from build123d import *

# Parameters (mm, degrees)
F0_W     = 63.5
F0_H     = 63.5
F0_W_2   = 50.8
F0_H_2   = 50.8
F1_DEPTH = 165.1
F3_R     = 6.477
F4_DEPTH = 25.4
F6_DEPTH = 25.4
F7_R     = 6.35
F8_DEPTH = 63.501


# Not quite as in the source:
# - ends of sketch curves that miss each other by under 0.0002 mm in the source are joined


with BuildPart() as f1:
    # F0 (on Top) → F1 (new body, symmetric)
    with BuildSketch(Plane.XY):
        Rectangle(F0_W, F0_H)
        Rectangle(F0_W_2, F0_H_2, mode=Mode.SUBTRACT)
    extrude(amount=F1_DEPTH, both=True)

    # F3 (on face) → F4 (cut)
    with BuildSketch(Plane.YZ.offset(31.75)):
        with Locations((0, 146.05)):
            Circle(F3_R)
        with BuildLine():
            ThreePointArc((10.1385245046, 129.1766616857), (14.6288058895, 132.8781640138), (17.8406687878, 137.7307595176))
            ThreePointArc((17.8406687878, 137.7307595176), (19.4934269332, 143.3103775076), (19.4426449846, 149.1294124443))
            ThreePointArc((19.4426449846, 149.1294124443), (15.0835370951, 152.2964897102), (11.9164598293, 147.9373818207))
            ThreePointArc((11.9164598293, 147.9373818207), (11.9475842494, 144.3708765369), (10.9346034506, 140.9511106721))
            ThreePointArc((10.9346034506, 140.9511106721), (8.9660423194, 137.9769392343), (6.2139343738, 135.708276517))
            ThreePointArc((6.2139343738, 135.708276517), (4.9104220235, 130.4801740359), (10.1385245046, 129.1766616857))
        make_face()
        with BuildLine():
            ThreePointArc((-10.1385245046, 129.1766616857), (-4.9104220235, 130.4801740359), (-6.2139343738, 135.708276517))
            ThreePointArc((-6.2139343738, 135.708276517), (-8.9660423194, 137.9769392343), (-10.9346034506, 140.9511106721))
            ThreePointArc((-10.9346034506, 140.9511106721), (-11.9475842494, 144.3708765369), (-11.9164598293, 147.9373818207))
            ThreePointArc((-11.9164598293, 147.9373818207), (-15.0835370951, 152.2964897102), (-19.4426449846, 149.1294124443))
            ThreePointArc((-19.4426449846, 149.1294124443), (-19.4934269332, 143.3103775076), (-17.8406687878, 137.7307595176))
            ThreePointArc((-17.8406687878, 137.7307595176), (-14.6288058895, 132.8781640138), (-10.1385245046, 129.1766616857))
        make_face()
    extrude(amount=-F4_DEPTH, mode=Mode.SUBTRACT)

    # F5 (on face) → F6 (cut)
    with BuildSketch(Plane(origin=(-31.75, 0, 0), x_dir=(0, -1, 0), z_dir=(-1, 0, 0))):
        with BuildLine():
            ThreePointArc((-3.1401119103, 140.3850881569), (3.2873259769, 140.4692279278), (6.477, 146.05))
            ThreePointArc((6.477, 146.05), (-3.2873259769, 151.6307720722), (-3.1401119103, 140.3850881569))
        make_face()
        with BuildLine():
            ThreePointArc((-5.7913527214, 132.1654121492), (-6.0549491708, 133.1322727306), (-6.7727903948, 133.8315626913))
            ThreePointArc((-6.7727903948, 133.8315626913), (-9.3377562721, 131.1985515677), (-5.7913527214, 132.1654121492))
        make_face()
        with BuildLine():
            ThreePointArc((3.1226517792, 134.3961049058), (0.4285749428, 129.7298269458), (5.0948529028, 127.0357501095))
            ThreePointArc((5.0948529028, 127.0357501095), (17.8406687878, 137.7307595176), (17.8406687878, 154.3692404824))
            ThreePointArc((17.8406687878, 154.3692404824), (12.777460542, 156.2120975737), (10.9346034506, 151.1488893279))
            ThreePointArc((10.9346034506, 151.1488893279), (10.9346034506, 140.9511106721), (3.1226517792, 134.3961049058))
        make_face()
    extrude(amount=-F6_DEPTH, mode=Mode.SUBTRACT)

    # F7 (on face) → F8 (cut, through all)
    with BuildSketch(Plane.YZ.offset(31.75)):
        with BuildLine():
            ThreePointArc((-8.89, 107.949999693), (-15.239999693, 101.6), (-8.89, 95.250000307))
            ThreePointArc((-8.89, 95.250000307), (3.81, 82.55), (-8.89, 69.85))
            ThreePointArc((-8.89, 69.85), (-15.239999693, 63.5), (-8.89, 57.150000307))
            ThreePointArc((-8.89, 57.150000307), (16.509999693, 82.55), (-8.89, 107.949999693))
        make_face()
        with BuildLine():
            ThreePointArc((8.89, 3.07e-07), (15.239999693, 6.35), (8.89, 12.699999693))
            ThreePointArc((8.89, 12.699999693), (-3.81, 25.4), (8.89, 38.1))
            ThreePointArc((8.89, 38.1), (15.24, 44.45), (8.89, 50.8))
            ThreePointArc((8.89, 50.8), (-16.509999693, 25.4), (8.89, 3.07e-07))
        make_face()
        with BuildLine():
            ThreePointArc((-8.89, -6.350000307), (-15.239999693, -12.7), (-8.89, -19.049999693))
            ThreePointArc((-8.89, -19.049999693), (3.81, -31.75), (-8.89, -44.45))
            ThreePointArc((-8.89, -44.45), (-15.239999693, -50.8), (-8.89, -57.149999693))
            ThreePointArc((-8.89, -57.149999693), (16.509999693, -31.75), (-8.89, -6.350000307))
        make_face()
        with BuildLine():
            ThreePointArc((8.89, -114.299999693), (15.239999693, -107.95), (8.89, -101.600000307))
            ThreePointArc((8.89, -101.600000307), (-3.81, -88.9), (8.89, -76.2))
            ThreePointArc((8.89, -76.2), (15.24, -69.85), (8.89, -63.5))
            ThreePointArc((8.89, -63.5), (-16.509999693, -88.9), (8.89, -114.299999693))
        make_face()
        with Locations((-8.89, 82.55)):
            Circle(F7_R)
        with Locations((8.89, 25.4)):
            Circle(F7_R)
        with Locations((8.89, -88.9)):
            Circle(F7_R)
        with Locations((-8.89, -31.75)):
            Circle(F7_R)
    extrude(amount=-F8_DEPTH, mode=Mode.SUBTRACT)


solid = f1.part
Geometry: final body of the model. Coordinates: model frame, mm. A direction names the side the tool comes from. Coordinates: 2 decimals unless noted, no trailing zeros. Loops run counter-clockwise (first coordinate to the right, second up) from the corner with the lowest first, then second, coordinate; pieces in that order, holes last. Notation, with made-up numbers: (69, -17.75) - (97, -17.75) arc R28 cw to (97, 19.25) - close; hole circle Ø5 at (59.25, -18). An arc over 180 degrees is marked (long way). One line per question, with ' | ' between items. Start each with the question number.
(1) Draft query along Z for faces 1 (the flat face through (25.4, -6, 2)), 2 (the flat face through (-29, 0, -165.1)), 3 (the cylindrical face through (-28.53, -15.24, -12.56)). Return one class per face: +Z half, -Z half, draft (parallel to the pull), parting line (faces both ways), or undercut.
(2) Cut plane B-B on x = 22. Output: boundary loops of the cut face in (y, z).
(3) Cut plane D-D on z = -106.5. Output: boundary loops of the cut face in (x, y), and give its area (3 significant figures).
(4) Reachability of faces 4 (the cylindrical face through (-28.619, -12.854, 156.247)), 5 (the flat face through (0, -31.75, 2)), 6 (the cylindrical face through (28.619, -3.807, -89.179)) from +Z, -Z, +X, -X, +Y, -Y: full face, straight path, thin tool, end or side. Return the list, or none.
(5) Cut plane A-A on z = 82.55. Output: boundary loops of the cut face in (x, y).
(6) Ray query, L1, parallel to Y at x = -29, z = 146; L2, parallel to X at y = 2, z = -83.5. Return the intervals inside material, ascending. Write a range as from..to.
Here are the results:
1) face 1: draft | face 2: -Z half | face 3: undercut
2) outline: (-31.75, -165.1) - (-25.4, -165.1) - (-25.4, 165.1) - (-31.75, 165.1) - close; (25.4, -165.1) - (31.75, -165.1) - (31.75, 165.1) - (25.4, 165.1) - close
3) outline: (-31.75, -31.75) - (31.75, -31.75) - (31.75, -9.42) - (25.4, -9.42) - (25.4, -25.4) - (-25.4, -25.4) - (-25.4, -9.42) - (-31.75, -9.42) - close; (-31.75, 15.07) - (-25.4, 15.07) - (-25.4, 25.4) - (25.4, 25.4) - (25.4, 15.07) - (31.75, 15.07) - (31.75, 31.75) - (-31.75, 31.75) - close | area: 1,140 mm²
4) face 4: -X | face 5: +Z, -Z, +X, -X, -Y | face 6: +X, -X
5) outline: (-31.75, -31.75) - (31.75, -31.75) - (31.75, -15.24) - (25.4, -15.24) - (25.4, -25.4) - (-25.4, -25.4) - (-25.4, -15.24) - (-31.75, -15.24) - close; (-31.75, -2.54) - (-25.4, -2.54) - (-25.4, 3.81) - (-31.75, 3.81) - close; (-31.75, 16.51) - (-25.4, 16.51) - (-25.4, 25.4) - (25.4, 25.4) - (25.4, 16.51) - (31.75, 16.51) - (31.75, 31.75) - (-31.75, 31.75) - close; (25.4, -2.54) - (31.75, -2.54) - (31.75, 3.81) - (25.4, 3.81) - close
6) L1: -31.75..-19.68, -12.06..-6.48, 6.48..31.75 | L2: -31.75..-25.4, 25.4..31.75
